Can you work these out from the model? Positions are in its coordinate system, mm. A direction names the side the tool comes from. Round coordinates to 2 decimals unless told otherwise and drop trailing zeros. Loops run counter-clockwise (first coordinate to the right, second up) from the corner with the lowest first, then second, coordinate; pieces in that order, holes last. Notation, with made-up numbers: (3.25, -36.75) - (50.25, -36.75) arc R17 ccw to (50.25, -23.75) - close; hole circle Ø6 at (72.25, -28). An arc over 180 degrees is marked (long way). Answer as CSV lines item,"result".
```python
from build123d import *

# Parameters (mm, degrees)
CHAMFER1_SIZE      = 1.190625
CHAMFER2_SIZE      = 0.619125
CUT_EXTRUDE2_DEPTH = 3.96875


with BuildPart() as part:
    # Sketch1 → Revolve1 (revolve)
    with BuildSketch(Plane(origin=(0, 0, 0), x_dir=(0, 0, -1), z_dir=(1, 0, 0))):
        Polygon((0, 9.525), (7.9375, 9.525), (7.9375, 6.35), (46.0375, 6.35), (46.0375, 4.7625), (61.9125, 4.7625), (61.9125, 0), (0, 0), align=None)
    revolve(axis=Axis((0, 0, -61.9125), (0, 0, 1)))

    # Sketch5 → Cut-Revolve1 (revolve, cut)
    with BuildSketch(Plane(origin=(0, 0, 0), x_dir=(0, 0, -1), z_dir=(1, 0, 0))):
        with BuildLine():
            Line((46.0375, 6.35), (51.8668, 6.35))
            Line((51.8668, 6.35), (49.2125, 3.6957))
            Line((49.2125, 3.6957), (47.1043, 3.6957))
            ThreePointArc((47.1043, 3.6957), (46.349958486, 4.008158486), (46.0375, 4.7625))
            Line((46.0375, 4.7625), (46.0375, 6.35))
        make_face()
    revolve(axis=Axis((0, 0, -61.9125), (0, 0, 1)), mode=Mode.SUBTRACT)

    # Chamfer1
    chamfer1_edges = [part.edges().sort_by_distance(p)[0] for p in [
        (0, -4.7625, -61.9125),
    ]]
    chamfer(chamfer1_edges, length=CHAMFER1_SIZE)

    # Chamfer2
    chamfer2_edges = [part.edges().sort_by_distance(p)[0] for p in [
        (0, -6.35, -46.0375),
        (0, -9.525, 0),
    ]]
    chamfer(chamfer2_edges, length=CHAMFER2_SIZE)

    # Sketch8 → Cut-Extrude2 (cut)
    with BuildSketch(Plane.XY):
        Polygon((3.175, 1.833087105), (0, 3.666174209), (-3.175, 1.833087105), (-3.175, -1.833087105), (0, -3.666174209), (3.175, -1.833087105), align=None)
    extrude(amount=-CUT_EXTRUDE2_DEPTH, mode=Mode.SUBTRACT)

    # Cut-Extrude4 cone 1 section (through the dimple's axis) → Cut-Extrude4 (revolve, cut)
    with BuildSketch(Plane(origin=(0, 0, 0), x_dir=(0, -1, 0), z_dir=(1, 0, 0))):
        Polygon((0, 0), (3.666174209, 0), (0, 3.666174209), align=None)
    revolve(axis=Axis((0, 0, 0), (0, 0, -1)), mode=Mode.SUBTRACT)


solid = part.part
```
Q1. If I drill on line 1 along Z through (x, y) = (-2.25, -2); line 2 along Z through (x, y) = (-1, -5); line 3 along X through (y, z) = (0.5, -48), over which ranges is the centre line in solid material (lowest first)? Write a range as [from, to].
Checks:
line 1,"[-61.91, -3.97]"
line 2,"[-46.04, 0]"
line 3,"[-3.66, 3.66]"
Q2. Imagine slicing it at B-B (z = -55.5). Write out the boundary of the cut face in (x, y) (1 decimal), then the cut area to 3 significant figures.
Checks:
outline,"circle Ø9.5 at (0, 0)"
area,"71.3 mm²"
Q3. Imagine slicing it at C-C (z = -44). Write out the boundary of the cut face in (x, y), then the cut area to 3 significant figures.
Checks:
outline,"circle Ø12.7 at (0, 0)"
area,"127 mm²"
Q4. We'd pull the mould along Z, two halves only. Please class faces 1 (the flat face through (0, 0, -3.969)), 2 (the cylindrical face through (3.61, -0.8, -48.14)), 3 (the flat face through (3.175, 0, -2)): pulls with the +Z half, pulls with the -Z half, needs draft (parallel to the pull), parting line crosses it, or undercut.
Checks:
face 1,"pulls with the +Z half"
face 2,"undercut"
face 3,"needs draft"
Q5. I'm going to push flat-ended pins straight in: pin 1 Ø5 at (y, z) = (2, -16) entering from +X; pin 2 Ø3 at (x, y) = (1, -0.5) entering from +Z; pin 3 Ø1.5 at (x, z) = (-3, -40) entering from -Y. Where does each tip first touch, or does it pass through?
Checks:
pin 1,"x = 6.35"
pin 2,"z = -3.97"
pin 3,"y = -5.94"
Q6. On a 3-axis mill with a long thin cutter (end or side, diameter ignored), from which of +Z, -Z, +X, -X, +Y, -Y can I reach the whole of each face in a straight line? I mean faces 4 (the cylindrical face through (6.2, -1.38, -26.94)), 5 (the flat face through (0, -4, 0)), 6 (the flat face through (-3.175, 0, -2)). Say none if no direction works.
Checks:
face 4,"-Z"
face 5,"+Z, +X, -X, +Y, -Y"
face 6,"+Z"
